from build123d import *

# Parameters (mm, degrees)
SKETCH_1_R      = 4.1
EXTRUDE_1_DEPTH = 4


with BuildPart() as part:
    # 草图1 → 凸台-拉伸1 (new body)
    with BuildSketch(Plane(origin=(0, 0, 0), x_dir=(1, 0, 0), z_dir=(0, 1, 0))):
        with BuildLine():
            Line((-2.083455003, 11.817750008), (50, 21))
            Line((50, 21), (131.330576007, 11.926003836))
            ThreePointArc((131.330576007, 11.926003836), (142, 0), (131.330576007, -11.926003836))
            Line((131.330576007, -11.926003836), (50, -21))
            Line((50, -21), (-2.083455003, -11.817750008))
            ThreePointArc((-2.083455003, -11.817750008), (-12, 0), (-2.083455003, 11.817750008))
        make_face()
        with Locations(Location((0, 0, 0), (0, 0, 270))):
            Circle(SKETCH_1_R, mode=Mode.SUBTRACT)
        with Locations(Location((50, 0, 0), (0, 0, 270))):
            Circle(SKETCH_1_R, mode=Mode.SUBTRACT)
        with Locations(Location((130, 0, 0), (0, 0, 270))):
            Circle(SKETCH_1_R, mode=Mode.SUBTRACT)
    extrude(amount=EXTRUDE_1_DEPTH)

    # 圆角1
    # a fillet whose section is not a circle: 40 mm, written as the material it takes off along each edge
    with BuildSketch(Plane(origin=(50, -14.378648939, 21), x_dir=(0.9938336529777407, 0, -0.11088133390665686), z_dir=(0, 1, 0)), Plane(origin=(50, -14.378648939, -21), x_dir=(-0.9848125006580993, 0, 0.17362125027640163), z_dir=(0, 1, 0))) as fillet_1_piece_1:
        with BuildLine():
            add(Edge.make_bspline([(5.751459576, 0), (4.676371086, 0), (3.601282597, 0), (1.210344489, 0.06897002), (-1.141879394, 0.407188034), (-3.455389054, 1.014654044), (-4.486924042, 1.317558038), (-5.518459029, 1.620462032)], knots=[0, 0, 0, 0, 0, 0, 0.5, 0.5, 1, 1, 1, 1, 1, 1], degree=5))
            Line((-5.518459029, 1.620462032), (0, 0))
            Line((0, 0), (5.751459576, 0))
        make_face()
    extrude(amount=32.757297879, mode=Mode.SUBTRACT)


solid = part.part
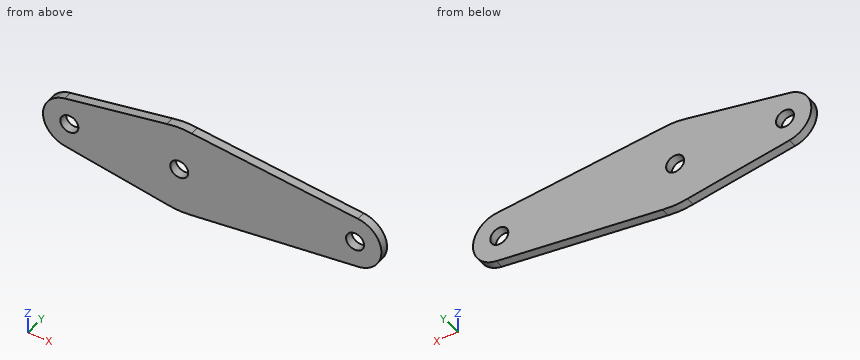
For this review, take the finished solid that the model builds, in its own axes (mm). Round coordinates to 2 decimals unless told otherwise and drop trailing zeros. Loops run counter-clockwise (first coordinate to the right, second up) from the corner with the lowest first, then second, coordinate; pieces in that order, holes last. Notation, with made-up numbers: (-35.5, 77.25) - (16.5, 77.25) arc R14 ccw to (16.5, 96.25) - close; hole circle Ø2 at (75.5, -13.5). An arc over 180 degrees is marked (long way). Put each result on its own line as item: value. Start each with the question number.
1. Consider section B-B on x = 0. State the section outline as (y, z) points, plus the area to 3 significant figures.
2. Consider section D-D on x = 64.5. State the section outline as (y, z) points.
3. For probe 1 along X at (y, z) = (1, 0); probe 2 along X at (y, z) = (2.8, 1); probe 3 along Z at (x, y) = (49, 1.1), list the stretches that pass through material, from the lowest coordinate up. Write a range as [from, to].
4. Insertion check: P1, Ø1.5, axis at y = 1, z = 5, coming from the -X side. The pin has a flat end and moves straight along its axis. Give the tip position at first contact, or say it passes through.
5. Consider section C-C on y = 3.3. State how many separate pieces and enclosed holes the cut face has, plus the area to 3 significant figures.
6. Consider section A-A on z = 0. State the section outline as (x, y) points.
Result sheet:
1. outline: (0, -12.19) - (4, -12.19) - (4, -4.1) - (0, -4.1) - close; (0, 4.1) - (4, 4.1) - (4, 12.19) - (0, 12.19) - close
1. area: 64.7 mm^2
2. outline: (0, -19.38) - (4, -19.38) - (4, 19.38) - (0, 19.38) - close
3. probe 1: [-12, -4.1], [4.1, 45.9], [54.1, 125.9], [134.1, 142]
3. probe 2: [-11.96, -3.98], [3.98, 46.02], [53.98, 126.02], [133.98, 141.96]
3. probe 3: [-20.64, -3.98], [3.98, 20.64]
4. P1: x = -11.22
5. separate pieces: 1
5. enclosed holes: 3
5. area: 4,600 mm^2
6. outline: (-12, 0) - (-4.1, 0) - (-4.1, 4) - (-12, 4) - close; (4.1, 0) - (45.9, 0) - (45.9, 4) - (4.1, 4) - close; (54.1, 0) - (125.9, 0) - (125.9, 4) - (54.1, 4) - close; (134.1, 0) - (142, 0) - (142, 4) - (134.1, 4) - close
